For this review, use the dimensioned drawing (mm, ordinates from the lowest corner) and the shaded views. Round coordinates to 2 decimals unless told otherwise and drop trailing zeros. Write each loop counter-clockwise with the first axis right and the second up, starting at its lowest first coordinate (ties: lowest second). Pieces come first, ordered by that corner, then holes. Notation, with made-up numbers: (-15.75, 84.5) -> (42.25, 84.5) arc R17 cw to (42.25, 104.5) -> close; hole circle Ø10 at (37, -25). An arc over 180 degrees is marked (long way). Answer as CSV lines item,"result". Start each with the question number.
Item 1: Wall thickness on probe 1 along Y at (x, z) = (25, 7); probe 2 along Y at (x, z) = (22.5, 4.5); probe 3 along X at (y, z) = (66, 1): over which ranges is each line inside the solid? List them lowest first. Write a range as from..to.
Item 2: Take a section at C-C on z = 5. Give the boundary of the cut face in (x, y).
Item 3: Take a section at B-B on x = 23. Give the boundary of the cut face in (y, z), then the cut area to 3 significant figures.
Item 4: Mouldability with a two-part tool opening along Y and no side actions: class the marked faces 1, 2 and 3 as +Y half, -Y half, draft (parallel to the pull), parting line (faces both ways), or undercut.
Item 5: Take a section at A-A on y = 65. Give the boundary of the cut face in (x, z).
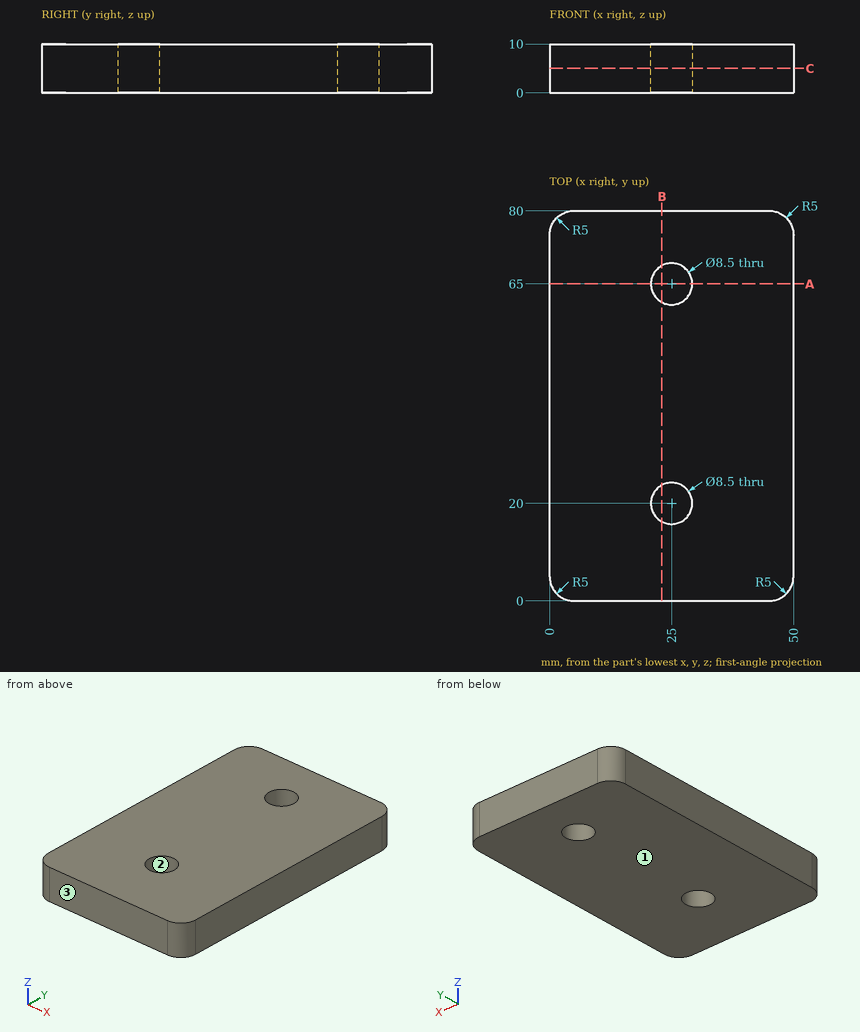
Output values:
1,probe 1,"y = 0..15.75, 24.25..60.75, 69.25..80"
1,probe 2,"y = 0..16.56, 23.44..61.56, 68.44..80"
1,probe 3,"x = 0..20.87, 29.13..50"
2,outline,"(0, 5) arc R5 ccw to (5, 0) -> (45, 0) arc R5 ccw to (50, 5) -> (50, 75) arc R5 ccw to (45, 80) -> (5, 80) arc R5 ccw to (0, 75) -> close; hole circle Ø8.5 at (25, 20); hole circle Ø8.5 at (25, 65)"
3,outline,"(0, 0) -> (16.25, 0) -> (16.25, 10) -> (0, 10) -> close; (23.75, 0) -> (61.25, 0) -> (61.25, 10) -> (23.75, 10) -> close; (68.75, 0) -> (80, 0) -> (80, 10) -> (68.75, 10) -> close"
3,area,"650 mm^2"
4,face 1,"draft"
4,face 2,"undercut"
4,face 3,"-Y half"
5,outline,"(0, 0) -> (20.75, 0) -> (20.75, 10) -> (0, 10) -> close; (29.25, 0) -> (50, 0) -> (50, 10) -> (29.25, 10) -> close"
